```python
from build123d import *

# Parameters (mm, degrees)
F1_DEPTH       = 12.7
F2_R           = 6.35
F4_DEPTH       = 6.35
F6_D           = 4.7752
F8_D           = 5.1054
F8_CBORE_D     = 9.4742
F8_CBORE_DEPTH = 4.826


with BuildPart() as f1:
    # F0 (on Front) → F1 (new body)
    with BuildSketch(Plane.XZ):
        with BuildLine():
            Line((52.387601, 42.861543), (-52.387399, 42.8625))
            ThreePointArc((-52.387399, 42.8625), (-63.5, 31.750051), (-52.3875, 20.6375))
            Line((-52.3875, 20.6375), (-39.6875, 20.6375))
            Line((-39.6875, 20.6375), (-39.6875, -20.6375))
            Line((-39.6875, -20.6375), (-52.533336, -20.6375))
            ThreePointArc((-52.533336, -20.6375), (-63.499761, -31.821912), (-52.387601, -42.861543))
            Line((-52.387601, -42.861543), (52.387399, -42.8625))
            ThreePointArc((52.387399, -42.8625), (63.5, -31.750051), (52.3875, -20.6375))
            Line((52.3875, -20.6375), (39.6875, -20.6375))
            Line((39.6875, -20.6375), (39.6875, 20.6375))
            Line((39.6875, 20.6375), (52.533336, 20.6375))
            ThreePointArc((52.533336, 20.6375), (63.499761, 31.821912), (52.387601, 42.861543))
        make_face()
    extrude(amount=F1_DEPTH)

    # F2
    f2_edges = [f1.edges().sort_by_distance(p)[0] for p in [
        (-39.6875, -6.35, 20.6375),
        (-39.6875, -6.35, -20.6375),
        (39.6875, -6.35, 20.6375),
        (39.6875, -6.35, -20.6375),
    ]]
    fillet(f2_edges, radius=F2_R)

    # F3 (on face) → F4 (join)
    with BuildSketch(Plane.XZ.offset(12.7)):
        Polygon((-38.1, -42.861674), (38.1, -42.86237), (38.1, 42.861674), (-38.1, 42.86237), align=None)
        Polygon((-38.1, 42.86237), (38.1, 42.861674), (38.1, 42.8625), (-38.1, 42.8625), align=None)
    extrude(amount=F4_DEPTH)

    # F6 (through all)
    with Locations(Plane.XZ.offset(12.7)):
        with Locations((-52.3875, 31.75), (52.3875, 31.75), (52.3875, -31.7373), (-52.3875, -31.7373)):
            Hole(F6_D / 2)

    # F8 (through all)
    with Locations(Plane(origin=(0, 0, 0), x_dir=(-1, 0, 0), z_dir=(0, 1, 0))):
        with Locations((-33.3375, 36.487274), (33.3375, 36.487883), (33.3375, -9.968717), (-33.3375, -9.969326)):
            CounterBoreHole(F8_D / 2, F8_CBORE_D / 2, F8_CBORE_DEPTH)


solid = f1.part
```
Verification items for the finished model (mm, model axes). A direction names the side the tool comes from. Coordinates: 2 decimals unless noted, no trailing zeros. Order: outer loops, then holes, each group sorted by start corner. A loop starts at its lowest first (then second) coordinate and runs counter-clockwise, first axis right, second up. Notation, with made-up numbers: (9, 87.25) -> (33, 87.25) arc R29 cw to (33, 116.25) -> close; hole circle Ø7 at (52, 27). An arc over 180 degrees is marked (long way). Answer as CSV lines item,"result". Start each with the question number.
1) Set-up check for faces 1 (the face through (-49, -6, 20.638)), 2 (the face through (37.097, -2.379, 33.605)), 3 (the face through (41.6, -6.44, -18.83)): record each of +Z, -Z, +X, -X, +Y, -Y from which the full face is reachable in a straight line by a thin tool's end or side.
2) Cross-section at C-C, the plane x = -34. Give the number of separate pieces and of enclosed holes in the cut face, then the cut area to 3 significant figures.
3) Cross-section at B-B, the plane z = 2. Record the boundary of the cut face in (x, y), then the cut area to 3 significant figures.
4) Cross-section at A-A, the plane x = 42.5. Record the boundary of the cut face in (y, z).
5) Release check for a two-part mould opening along Z. For faces 4 (the face through (-41.5, -6.44, -18.73)), 5 (the face through (-38.1, -16, 1)) record: released by +Z, released by -Z, zero draft, split by the parting line, or undercut.
6) Gauge pin test, flat ends, axial feed: pin 1 Ø6 at (x, z) = (-33.34, 36.49) entering from +Y; pin 2 Ø4.5 at (x, z) = (33.34, 36.49) entering from -Y; pin 3 Ø12.5 at (x, z) = (33.34, -9.97) entering from +Y; pin 4 Ø2 at (y, z) = (-14.5, -30.5) entering from +X. Record the tip position at first contact, or that the pin passes through.
7) Material ranges on L1, parallel to X at y = -7, z = -32; L2, parallel to X at y = -9.5, z = -8; L3, parallel to Z at x = -34, y = -12, recorded low to high. Write a range as [from, to].
8) Cross-section at D-D, the plane y = -16.5. Record the boundary of the cut face in (x, z).
Conclusion:
1,face 1,"-X, +Y, -Y"
1,face 2,"+Y"
1,face 3,"+X, +Y, -Y"
2,separate pieces,"3"
2,enclosed holes,"0"
2,area,"1,400 mm²"
3,outline,"(-39.69, -12.7) -> (-38.1, -12.7) -> (-38.1, -19.05) -> (38.1, -19.05) -> (38.1, -12.7) -> (39.69, -12.7) -> (39.69, 0) -> (-39.69, 0) -> close"
3,area,"1,490 mm²"
4,outline,"(-12.7, -42.86) -> (0, -42.86) -> (0, -19.56) -> (-12.7, -19.56) -> close; (-12.7, 19.56) -> (0, 19.56) -> (0, 42.86) -> (-12.7, 42.86) -> close"
5,face 4,"undercut"
5,face 5,"zero draft"
6,pin 1,"stops at y = -4.83"
6,pin 2,"passes through"
6,pin 3,"stops at y = 0"
6,pin 4,"stops at x = 38.1"
7,L1,"x = [-63.5, -54.76], [-50.01, 50.01], [54.76, 63.5]"
7,L2,"x = [-39.69, -34.96], [-31.71, 31.71], [34.96, 39.69]"
7,L3,"z = [-42.86, -12.43], [-7.5, 34.02], [38.95, 42.86]"
8,outline,"(-38.1, -42.86) -> (38.1, -42.86) -> (38.1, 42.86) -> (-38.1, 42.86) -> close; hole circle Ø5.11 at (-33.34, -9.97); hole circle Ø5.11 at (-33.34, 36.49); hole circle Ø5.11 at (33.34, -9.97); hole circle Ø5.11 at (33.34, 36.49)"
